Input: part model. Units: mm. Frame: model coordinates. Coordinates: 2 decimals unless noted, no trailing zeros. Order: outer loops, then holes, each group sorted by start corner. A loop starts at its lowest first (then second) coordinate and runs counter-clockwise, first axis right, second up. Notation, with made-up numbers: M 80.5,-14 L 125.5,-14 A19 ccw 125.5,-1 Z; hole C 47,41.5 d2. An arc over 180 degrees is marked long. Answer in a Markdown table with one row per item.
from build123d import *

# Parameters (mm, degrees)
F1_DEPTH     = 12.7
F2_DEPTH     = 12.192
F3_DEPTH     = 12.192
F4_DEPTH     = 12.192
F5_DEPTH     = 12.192
F6_DEPTH     = 12.192
F7_T4_ANGLE  = 291.9758344639
F7_T9_ANGLE  = 291.9758344639
F7_T14_ANGLE = 291.9758344639
F7_T19_ANGLE = 291.9758344639
F7_T24_ANGLE = 291.9758344639
F7_T29_ANGLE = 68.0241655361


# Not quite as in the source:
# - a fillet or chamfer that OpenCascade refuses, or shapes differently, is made with other operations: its cross-section is extruded or revolved along the edge and cut away or added


with BuildPart() as f1:
    # F0 (on Top) → F1 (new body)
    with BuildSketch(Plane.XY):
        Polygon((0, 24.0160203306), (-22.8405926309, 7.4213584194), (-14.1162625691, -19.4293685847), (14.1162625691, -19.4293685847), (22.8405926309, 7.4213584194), align=None)
    extrude(amount=F1_DEPTH)

    # F0 (on Top) → F2 (join)
    with BuildSketch(Plane.XY):
        with BuildLine():
            Line((-14.1162625691, -19.4293685847), (-22.8405926309, 7.4213584194))
            Line((-22.8405926309, 7.4213584194), (-28.2653771262, 11.4060885458))
            ThreePointArc((-28.2653771262, 11.4060885458), (-29.2974841135, -8.4076051653), (-17.9156944899, -24.6588379885))
            Line((-17.9156944899, -24.6588379885), (-14.1162625691, -19.4293685847))
        make_face()
    extrude(amount=F2_DEPTH)

    # F0 (on Top) → F3 (join)
    with BuildSketch(Plane.XY):
        with BuildLine():
            Line((-28.2653771262, 11.4060885458), (-22.8405926309, 7.4213584194))
            Line((-22.8405926309, 7.4213584194), (0, 24.0160203306))
            Line((0, 24.0160203306), (0, 30.48))
            ThreePointArc((0, 30.48), (-17.0495281625, 25.2654702992), (-28.2653771262, 11.4060885458))
        make_face()
    extrude(amount=F3_DEPTH)

    # F0 (on Top) → F4 (join)
    with BuildSketch(Plane.XY):
        with BuildLine():
            Line((0, 30.48), (0, 24.0160203306))
            Line((0, 24.0160203306), (22.8405926309, 7.4213584194))
            Line((22.8405926309, 7.4213584194), (28.2789000487, 11.3725200388))
            ThreePointArc((28.2789000487, 11.3725200388), (17.0645244472, 25.2553440957), (0, 30.48))
        make_face()
    extrude(amount=F4_DEPTH)

    # F0 (on Top) → F5 (join)
    with BuildSketch(Plane.XY):
        with BuildLine():
            Line((28.2789000487, 11.3725200388), (22.8405926309, 7.4213584194))
            Line((22.8405926309, 7.4213584194), (14.1162625691, -19.4293685847))
            Line((14.1162625691, -19.4293685847), (16.162839814, -25.8416912981))
            ThreePointArc((16.162839814, -25.8416912981), (26.6615243144, -14.7713750624), (30.48, 0))
            ThreePointArc((30.48, 0), (29.9246660256, 5.7917841169), (28.2789000487, 11.3725200388))
        make_face()
    extrude(amount=F5_DEPTH)

    # F0 (on Top) → F6 (join)
    with BuildSketch(Plane.XY):
        with BuildLine():
            Line((14.1162625691, -19.4293685847), (-14.1162625691, -19.4293685847))
            Line((-14.1162625691, -19.4293685847), (-17.9156944899, -24.6588379885))
            ThreePointArc((-17.9156944899, -24.6588379885), (-1.0573128046, -30.4616560553), (16.162839814, -25.8416912981))
            Line((16.162839814, -25.8416912981), (14.1162625691, -19.4293685847))
        make_face()
    extrude(amount=F6_DEPTH)

    # F7: fillet of radius 10.922 on 2 edges, made by hand


with BuildPart() as f7_tool2:
    # F7_s3 → F7_t4 (revolve)
    with BuildSketch(Plane(origin=(0, 0, 0), x_dir=(0, 0, 1), z_dir=(-0.8478245177, -0.5302768968, 0))):
        with BuildLine():
            ThreePointArc((12.192, -19.558), (8.9930202641, -27.2810202641), (1.27, -30.48))
            Line((1.27, -30.48), (12.192, -30.48))
            Line((12.192, -30.48), (12.192, -19.558))
        make_face()
    revolve(axis=Axis((0, 0, 12.192), (0, 0, 1)), revolution_arc=F7_T4_ANGLE)

    split(bisect_by=Plane.XZ.offset(19.4293685847), keep=Keep.TOP)


with BuildPart() as f1_1:
    add(f1.part)

    # F7_t1: cut F7_tool2
    add(f7_tool2.part, mode=Mode.SUBTRACT)


with BuildPart() as f7_tool7:
    # F7_s8 → F7_t9 (revolve)
    with BuildSketch(Plane(origin=(0, 0, 0), x_dir=(0, 0, 1), z_dir=(-0.8478245177, -0.5302768968, 0))):
        with BuildLine():
            ThreePointArc((12.192, -19.558), (8.9930202641, -27.2810202641), (1.27, -30.48))
            Line((1.27, -30.48), (12.192, -30.48))
            Line((12.192, -30.48), (12.192, -19.558))
        make_face()
    revolve(axis=Axis((0, 0, 12.192), (0, 0, 1)), revolution_arc=F7_T9_ANGLE)

    split(bisect_by=Plane(origin=(18.4784276, -6.0040050827, 0), x_dir=(0, 0, 1), z_dir=(0.9510565163, -0.3090169944, 0)), keep=Keep.TOP)


with BuildPart() as f1_2:
    add(f1_1.part)

    # F7_t6: cut F7_tool7
    add(f7_tool7.part, mode=Mode.SUBTRACT)


with BuildPart() as f7_tool12:
    # F7_s13 → F7_t14 (revolve)
    with BuildSketch(Plane(origin=(0, 0, 0), x_dir=(0, 0, 1), z_dir=(-0.8478245177, -0.5302768968, 0))):
        with BuildLine():
            ThreePointArc((12.192, -19.558), (8.9930202641, -27.2810202641), (1.27, -30.48))
            Line((1.27, -30.48), (12.192, -30.48))
            Line((12.192, -30.48), (12.192, -19.558))
        make_face()
    revolve(axis=Axis((0, 0, 12.192), (0, 0, 1)), revolution_arc=F7_T14_ANGLE)

    split(bisect_by=Plane(origin=(11.4202963155, 15.718689375, 0), x_dir=(0, 0, 1), z_dir=(0.5877852523, 0.8090169944, 0)), keep=Keep.TOP)


with BuildPart() as f1_3:
    add(f1_2.part)

    # F7_t11: cut F7_tool12
    add(f7_tool12.part, mode=Mode.SUBTRACT)


with BuildPart() as f7_tool17:
    # F7_s18 → F7_t19 (revolve)
    with BuildSketch(Plane(origin=(0, 0, 0), x_dir=(0, 0, 1), z_dir=(-0.8478245177, -0.5302768968, 0))):
        with BuildLine():
            ThreePointArc((12.192, -19.558), (8.9930202641, -27.2810202641), (1.27, -30.48))
            Line((1.27, -30.48), (12.192, -30.48))
            Line((12.192, -30.48), (12.192, -19.558))
        make_face()
    revolve(axis=Axis((0, 0, 12.192), (0, 0, 1)), revolution_arc=F7_T19_ANGLE)

    split(bisect_by=Plane(origin=(-11.4202963155, 15.718689375, 0), x_dir=(0, 0, 1), z_dir=(-0.5877852523, 0.8090169944, 0)), keep=Keep.TOP)


with BuildPart() as f1_4:
    add(f1_3.part)

    # F7_t16: cut F7_tool17
    add(f7_tool17.part, mode=Mode.SUBTRACT)


with BuildPart() as f7_tool22:
    # F7_s23 → F7_t24 (revolve)
    with BuildSketch(Plane(origin=(0, 0, 0), x_dir=(0, 0, 1), z_dir=(-0.8478245177, -0.5302768968, 0))):
        with BuildLine():
            ThreePointArc((12.192, -19.558), (8.9930202641, -27.2810202641), (1.27, -30.48))
            Line((1.27, -30.48), (12.192, -30.48))
            Line((12.192, -30.48), (12.192, -19.558))
        make_face()
    revolve(axis=Axis((0, 0, 12.192), (0, 0, 1)), revolution_arc=F7_T24_ANGLE)

    split(bisect_by=Plane(origin=(-18.4784276, -6.0040050827, 0), x_dir=(0, 0, 1), z_dir=(-0.9510565163, -0.3090169944, 0)), keep=Keep.TOP)


with BuildPart() as f1_5:
    add(f1_4.part)

    # F7_t21: cut F7_tool22
    add(f7_tool22.part, mode=Mode.SUBTRACT)


with BuildPart() as f7_tool27:
    # F7_s28 → F7_t29 (revolve)
    with BuildSketch(Plane(origin=(0, 0, 0), x_dir=(0, 0, 1), z_dir=(-0.8090169944, 0.5877852523, 0))):
        with BuildLine():
            ThreePointArc((12.192, -19.558), (8.9930202641, -27.2810202641), (1.27, -30.48))
            Line((1.27, -30.48), (12.192, -30.48))
            Line((12.192, -30.48), (12.192, -19.558))
        make_face()
    revolve(axis=Axis((0, 0, 12.192), (0, 0, 1)), revolution_arc=F7_T29_ANGLE)

    split(bisect_by=Plane.XZ.offset(19.4293685847), keep=Keep.TOP)


with BuildPart() as f1_6:
    add(f1_5.part)

    # F7_t26: cut F7_tool27
    add(f7_tool27.part, mode=Mode.SUBTRACT)


solid = f1_6.part
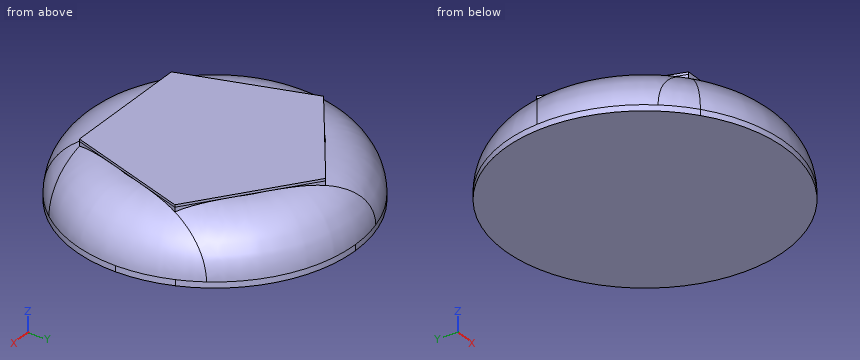
1) Cut plane A-A, the plane z = 7.75. Output: boundary loops of the cut face in (x, y).
Resolved:
| item | result |
|---|---|
| outline | C 0,0 d56.7 |
2) Contact query for flat-ended pins moving along their axis: pin 1 (2 mm diameter, centred on x = 12, y = 15.5, fed in from +Z); pin 2 (1.5 mm diameter, centred on x = 14, z = 2, fed in from +Y); pin 3 (3 mm diameter, centred on y = -20, z = 8, fed in from -X); pin 4 (3 mm diameter, centred on y = 3.5, z = 5.5, fed in from +X). Output: stop coordinate, or through.
Resolved:
| item | result |
|---|---|
| pin 1 | stops at z = 12.7 |
| pin 2 | stops at y = 27.43 |
| pin 3 | stops at x = -21.82 |
| pin 4 | stops at x = 29.96 |
3) Material intervals for probe 1 along X at (y, z) = (-17, 6.5); probe 2 along X at (y, z) = (9.5, 10.5); probe 3 along Z at (x, y) = (20, -4.5), sorted ascending.
Resolved:
| item | result |
|---|---|
| probe 1 | x = -23.68 to 23.68 |
| probe 2 | x = -23.55 to 23.55 |
| probe 3 | z = 0 to 12.15 |
